```python
from build123d import *

# Parameters (mm, degrees)
SKETCH1_R                = 2.55
BOSS_EXTRUDE1_DEPTH      = 24
BOSS_EXTRUDE2_DEPTH      = 5
BOSS_EXTRUDE3_DEPTH      = 5
BOSS_EXTRUDE5_DEPTH      = 7.5
BOSS_EXTRUDE5_DEPTH_BACK = 7.5
SKETCH4_W                = 15
SKETCH4_H                = 14
SKETCH9_R                = 4.986373578
CUT_EXTRUDE2_DEPTH       = 16.5


with BuildPart() as part:
    # Sketch1 → Boss-Extrude1 (new body)
    with BuildSketch(Plane.XY):
        Circle(SKETCH1_R)
    extrude(amount=BOSS_EXTRUDE1_DEPTH)

    # Sketch2 → Boss-Extrude2 (add)
    with BuildSketch(Plane.XY.offset(24)):
        Polygon((3.262188456, 0), (1.631094228, 2.825138074), (-1.631094228, 2.825138074), (-3.262188456, 0), (-1.631094228, -2.825138074), (1.631094228, -2.825138074), align=None)
    extrude(amount=BOSS_EXTRUDE2_DEPTH)

    # Sketch3 → Boss-Extrude3 (add)
    with BuildSketch(Plane(origin=(0, 0, 0), x_dir=(-1, 0, 0), z_dir=(0, 0, -1))):
        Polygon((3.262188456, 0), (1.631094228, 2.825138074), (-1.631094228, 2.825138074), (-3.262188456, 0), (-1.631094228, -2.825138074), (1.631094228, -2.825138074), align=None)
    extrude(amount=BOSS_EXTRUDE3_DEPTH)

    # Sketch4 → Boss-Extrude5 (add, two sides: drawn at the far end of the back side and taken through both)
    with BuildSketch(Plane(origin=(0, 0, 0), x_dir=(1, 0, 0), z_dir=(0, 1, 0)).offset(-BOSS_EXTRUDE5_DEPTH_BACK)):
        with Locations((0.05, -12)):
            Rectangle(SKETCH4_W, SKETCH4_H)
    extrude(amount=BOSS_EXTRUDE5_DEPTH + BOSS_EXTRUDE5_DEPTH_BACK)

    # Sketch9 → Cut-Extrude2 (cut)
    with BuildSketch(Plane(origin=(0, 7.5, 0), x_dir=(1, 0, 0), z_dir=(0, 1, 0))):
        with Locations(Location((0.05, -12.031387259, 0), (0, 0, 270))):
            Circle(SKETCH9_R)
    extrude(amount=-CUT_EXTRUDE2_DEPTH, mode=Mode.SUBTRACT)


solid = part.part
```
Could you check a few things on this model? Use its own coordinates, in mm. A direction names the side the tool comes from. Round coordinates to 2 decimals unless told otherwise and drop trailing zeros. Write each loop counter-clockwise with the first axis right and the second up, starting at its lowest first coordinate (ties: lowest second). Pieces come first, ordered by that corner, then holes. Notation, with made-up numbers: M 22.5,57.25 L 66.5,57.25 A19 cw 66.5,77.25 Z; hole C 77,63.5 d10. An arc over 180 degrees is marked long. Answer in a Markdown table with one row per item. Add a question column.
Q1. On a 3-axis mill with a long thin cutter (end or side, diameter ignored), from which of +Z, -Z, +X, -X, +Y, -Y can I reach the whole of each face in a straight line? I mean faces 1 (the flat face through (2.435, 1.432, -2.465)), 2 (the flat face through (0, -2.825, 26)), 3 (the flat face through (0, 2.825, -2)), 4 (the flat face through (-2.46, 1.39, -2.46)), 5 (the flat face through (-2.435, -1.432, -2.465)). Say none if no direction works.
Q2. Imagine slicing it at A-A (x = 0.05). Please give me the cut outline in (y, z), then the cut area to 3 significant figures.
Q3. Imagine slicing it at D-D (z = -1). Please give me the cut outline in (x, y).
Q4. Imagine slicing it at C-C (y = -4.5). Please give me the cut outline in (x, z).
Q5. Will these pins go through, and if not, where does the flat tip stop? pin 1 Ø1.6 at (x, z) = (0.5, 26) entering from -Y; pin 2 Ø3.5 at (x, z) = (0.5, -2.5) entering from +Y; pin 3 Ø5 at (x, y) = (-5.5, -1.5) entering from -Z.
Q6. Imagine slicing it at B-B (z = 8.5). Please give me the cut outline in (x, y), then the cut area to 3 significant figures.
Q7. If I drill on line 1 (X direction, y = -4, z = 12); line 2 (Z direction, x = 0.25, y = -6.5); line 3 (Z direction, x = 3.25, y = -1.5), over which ranges is the centre line in solid material (lowest first)? Write a range as from..to.
Q8. If we mould it in two halves opening along Z, with no side actions, what happens to faces 6 (the cylindrical face through (1.18, -2.26, 21.46)), 7 (the flat face through (0, 0, 29)), 8 (the flat face through (0, 2.825, 26))? For each: +Z half, -Z half, draft (parallel to the pull), parting line (faces both ways), or undercut.
Values:
| question | item | result |
|---|---|---|
| 1 | face 1 | -Z, +X, +Y |
| 1 | face 2 | +Z, +X, -X, -Y |
| 1 | face 3 | -Z, +X, -X, +Y |
| 1 | face 4 | -Z, -X, +Y |
| 1 | face 5 | -Z, -X, -Y |
| 2 | outline | M -7.5,5 L -2.55,5 L -2.55,0 L -2.83,0 L -2.83,-5 L 2.83,-5 L 2.83,0 L 2.55,0 L 2.55,5 L 7.5,5 L 7.5,7.05 L -7.5,7.05 Z; M -7.5,17.02 L 7.5,17.02 L 7.5,19 L 2.55,19 L 2.55,24 L 2.83,24 L 2.83,29 L -2.83,29 L -2.83,24 L -2.55,24 L -2.55,19 L -7.5,19 Z |
| 2 | area | 168 mm^2 |
| 3 | outline | M -3.26,0 L -1.63,-2.83 L 1.63,-2.83 L 3.26,0 L 1.63,2.83 L -1.63,2.83 Z |
| 4 | outline | M -7.45,5 L 7.55,5 L 7.55,19 L -7.45,19 Z; hole C 0.05,12.03 d9.97 |
| 5 | pin 1 | y = -2.83 |
| 5 | pin 2 | y = 2.83 |
| 5 | pin 3 | z = 5 |
| 6 | outline | M -7.45,-7.5 L -3.47,-7.5 L -3.47,7.5 L -7.45,7.5 Z; M 3.57,-7.5 L 7.55,-7.5 L 7.55,7.5 L 3.57,7.5 Z |
| 6 | area | 119 mm^2 |
| 7 | line 1 | -7.45..-4.94, 5.04..7.55 |
| 7 | line 2 | 5..7.05, 17.01..19 |
| 7 | line 3 | 5..8.21, 15.86..19 |
| 8 | face 6 | undercut |
| 8 | face 7 | +Z half |
| 8 | face 8 | draft |
